CAD build for the part. Positions are in the model's coordinates, mm. A direction names the side the tool comes from. Coordinates: 2 decimals unless noted, no trailing zeros. Write each loop counter-clockwise with the first axis right and the second up, starting at its lowest first coordinate (ties: lowest second). Pieces come first, ordered by that corner, then holes. Notation, with made-up numbers: M 15,-30.5 L 33,-30.5 A16 ccw 33,-26.5 Z; hole C 77.5,-2.5 d7. An arc over 180 degrees is marked long. Put each result on its own line as item: value. Start each with the question number.
```python
from build123d import *

# Parameters (mm, degrees)
SKETCH2_R           = 5
BOSS_EXTRUDE1_DEPTH = 10
SKETCH3_R           = 10
SKETCH3_R_2         = 5
BOSS_EXTRUDE2_DEPTH = 76.2
BOSS_EXTRUDE3_START = 86.2
SKETCH2_2_R         = 5
BOSS_EXTRUDE3_DEPTH = 22
SKETCH5_R           = 65
BOSS_EXTRUDE4_DEPTH = 22
SKETCH6_R           = 55
CUT_EXTRUDE1_DEPTH  = 22


with BuildPart() as part:
    # Sketch2 → Boss-Extrude1 (new body)
    with BuildSketch(Plane.XY):
        with BuildLine():
            Line((-19.794866372, 2.857142857), (-9.897433186, 71.428571429))
            ThreePointArc((-9.897433186, 71.428571429), (0, 80), (9.897433186, 71.428571429))
            Line((9.897433186, 71.428571429), (19.794866372, 2.857142857))
            ThreePointArc((19.794866372, 2.857142857), (0, -20), (-19.794866372, 2.857142857))
        make_face()
        with Locations((0, 70)):
            Circle(SKETCH2_R, mode=Mode.SUBTRACT)
        with BuildLine():
            Line((-2.5, 9.682458366), (-2.5, 12))
            Line((-2.5, 12), (2.5, 12))
            Line((2.5, 12), (2.5, 9.682458366))
            ThreePointArc((2.5, 9.682458366), (0, -10), (-2.5, 9.682458366))
        make_face(mode=Mode.SUBTRACT)
    extrude(amount=BOSS_EXTRUDE1_DEPTH)

    # Sketch3 → Boss-Extrude2 (add)
    with BuildSketch(Plane.XY.offset(10)):
        with Locations(Location((0, 70, 0), (0, 0, 171.786789298))):
            Circle(SKETCH3_R)
        with Locations((0, 70)):
            Circle(SKETCH3_R_2, mode=Mode.SUBTRACT)
    extrude(amount=BOSS_EXTRUDE2_DEPTH)

    # Sketch2<2> → Boss-Extrude3 (add)
    with BuildSketch(Plane.XY.offset(BOSS_EXTRUDE3_START)):
        with BuildLine():
            Line((-19.794866372, 2.857142857), (-9.897433186, 71.428571429))
            ThreePointArc((-9.897433186, 71.428571429), (0, 80), (9.897433186, 71.428571429))
            Line((9.897433186, 71.428571429), (19.794866372, 2.857142857))
            ThreePointArc((19.794866372, 2.857142857), (0, -20), (-19.794866372, 2.857142857))
        make_face()
        with Locations((0, 70)):
            Circle(SKETCH2_2_R, mode=Mode.SUBTRACT)
        with BuildLine():
            Line((-2.5, 9.682458366), (-2.5, 12))
            Line((-2.5, 12), (2.5, 12))
            Line((2.5, 12), (2.5, 9.682458366))
            ThreePointArc((2.5, 9.682458366), (0, -10), (-2.5, 9.682458366))
        make_face(mode=Mode.SUBTRACT)
    extrude(amount=BOSS_EXTRUDE3_DEPTH)

    # Sketch5 → Boss-Extrude4 (add)
    with BuildSketch(Plane.XY.offset(108.2)):
        Circle(SKETCH5_R)
    extrude(amount=-BOSS_EXTRUDE4_DEPTH)

    # Sketch6 → Cut-Extrude1 (cut)
    with BuildSketch(Plane.XY.offset(108.2)):
        Circle(SKETCH6_R)
    extrude(amount=-CUT_EXTRUDE1_DEPTH, mode=Mode.SUBTRACT)


solid = part.part
```
(1) Which spindle directions (+Z, -Z, +X, -X, +Y, -Y) get a long thin tool onto all of the face, cutting with end or side? Do faces 1 (the face through (0, 12, 5)), 2 (the face through (0, 56, 108.2)). Say none if no direction does.
(2) Slice it at D-D, the plane y = 0. Write the cut outline in (x, z), then the cut area to 3 significant figures.
(3) Drop flat-ended pins along their axis: pin 1 (1.5 mm diameter, centred on x = 0, z = 5, fed in from -Y); pin 2 (3 mm diameter, centred on x = -14.5, y = 49, fed in from +Z); pin 3 (2.5 mm diameter, centred on y = 10.5, z = 5.5, fed in from -X); pin 4 (9 mm diameter, centred on x = 0, y = 70, fed in from -Z). Give the stop position or say it passes through.
(4) Slice it at A-A, the plane x = 0. Write the cut outline in (y, z).
(5) Slice it at C-C, the plane x = -14. Write the cut outline in (y, z), then the cut area to 3 significant figures.
(6) Slice it at B-B, the plane y = -23.5. Write the cut outline in (x, z), then the cut area to 3 significant figures.
(7) Two-plate mould, pull along X, no slides. Class faces 3 (the face through (-11.923, -53.692, 97.354)), 4 (the face through (-14.915, 36.663, 4.93)), 5 (the face through (10.42, 67.8, 97.05)): +X half, -X half, draft (parallel to the pull), parting line (faces both ways), or undercut.
(8) Drill centre lines: line 1 (X direction, y = 70, z = 30.5); line 2 (Z direction, x = -10, y = 41); line 3 (Y direction, x = 0, z = 25). Where is each one in solid material? Low to high. Write a range as [from, to].
Result set:
1. face 1: +Z, -Z
1. face 2: +Z, +X, -X, +Y, -Y
2. outline: M -65,86.2 L -55,86.2 L -55,108.2 L -65,108.2 Z; M -20,0 L -10,0 L -10,10 L -20,10 Z; M 10,0 L 20,0 L 20,10 L 10,10 Z; M 55,86.2 L 65,86.2 L 65,108.2 L 55,108.2 Z
2. area: 640 mm^2
3. pin 1: stops at y = -20
3. pin 2: stops at z = 10
3. pin 3: stops at x = -18.87
3. pin 4: passes through
4. outline: M -65,86.2 L -55,86.2 L -55,108.2 L -65,108.2 Z; M -20,0 L -10,0 L -10,10 L -20,10 Z; M 12,0 L 65,0 L 65,108.2 L 55,108.2 L 55,86.2 L 60,86.2 L 60,10 L 12,10 Z; M 75,0 L 80,0 L 80,108.2 L 75,108.2 Z
5. outline: M -63.47,86.2 L -53.19,86.2 L -53.19,108.2 L -63.47,108.2 Z; M -14.28,0 L 43.01,0 L 43.01,10 L -14.28,10 Z; M 53.19,86.2 L 63.47,86.2 L 63.47,108.2 L 53.19,108.2 Z
5. area: 1,030 mm^2
6. outline: M -60.6,86.2 L -49.73,86.2 L -49.73,108.2 L -60.6,108.2 Z; M 49.73,86.2 L 60.6,86.2 L 60.6,108.2 L 49.73,108.2 Z
6. area: 479 mm^2
7. face 3: undercut
7. face 4: -X half
7. face 5: +X half
8. line 1: x = [-10, -5], [5, 10]
8. line 2: z = [0, 10]
8. line 3: y = [60, 65], [75, 80]
